The model under review builds one solid part; all positions refer to its coordinate system, in mm. Face numbers are marked on the shaded views. A direction names the side the tool comes from. Round coordinates to 2 decimals unless told otherwise and drop trailing zeros. Order: outer loops, then holes, each group sorted by start corner. A loop starts at its lowest first (then second) coordinate and runs counter-clockwise, first axis right, second up. Notation, with made-up numbers: M 79.25,37 L 124.25,37 A30 ccw 124.25,76 Z; hole C 49,68 d11. An arc over 180 degrees is marked long. Answer as a JSON object with one key per item and string values. Group by question number.
1. Mouldability with a two-part tool opening along Y and no side actions: class the marked faces 1, 2, 3 and 4 as released by +Y, released by -Y, zero draft, split by the parting line, or undercut.
2. Add section B-B on x = 32.5. State the section outline as (y, z) points (3 decimals), and give its area (3 significant figures).
3. Add section A-A on y = -14.5. State the section outline as (x, z) points, and give its area (3 significant figures).
4. Add section D-D on z = 3.25. Give the number of separate pieces and of enclosed holes in the cut face, and give its area (3 significant figures).
5. To check wall thickness, follow probe 1 along X at (y, z) = (-4, 5.25) (3 decimals); probe 2 along X at (y, z) = (8, 5.5) (3 decimals); probe 3 along Y at (x, z) = (34, 5.75) (3 decimals). State the ranges of each line that lie inside material, in increasing order. Write a range as [from, to].
6. Machinability: for the marked faces 5, 6 and 7, which of the approach directions +Z, -Z, +X, -X, +Y, -Y give a long, thin tool a straight path to every point of the face, cutting with its end or side? Answer none if there is none.
7. Add section C-C on y = -7.5. State the section outline as (x, z) points (3 decimals).
8. Clearance check with flat-ended pins moving along their axes: P1, Ø1, axis at y = -2, z = 3.5, coming from the +X side; P2, Ø1, axis at x = 27, z = 2.5, coming from the -Y side (3 decimals); P3, Ø2, axis at x = 29.5, z = 3.5, coming from the +Y side (3 decimals). State where each tip first meets the part, or that it passes through.
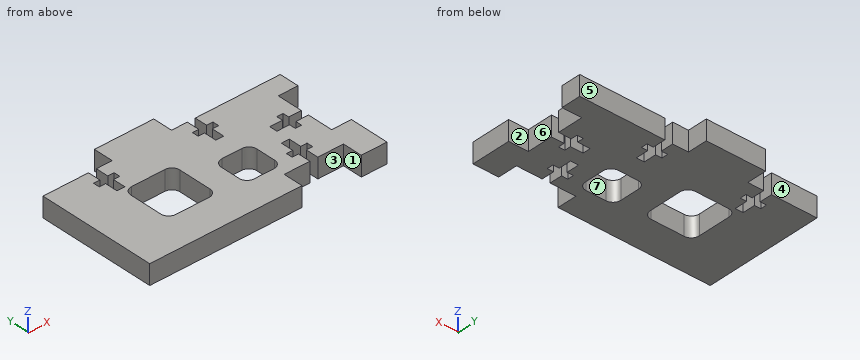
```python
from build123d import *

# Parameters (mm, degrees)
SKETCH1_W               = 76.2
SKETCH1_H               = 31.75
BOSS_EXTRUDE1_DEPTH     = 6.35
SKETCH2_W               = 19.05
SKETCH2_H               = 6.35
BOSS_EXTRUDE2_DEPTH     = 6.35
CUT_EXTRUDE1_DEPTH      = 6.35
CUT_EXTRUDE4_DEPTH      = 6.35
SKETCH5_W               = 76.2
SKETCH5_H               = 6.35
BOSS_EXTRUDE3_DEPTH     = 6.35
CUT_EXTRUDE7_DEPTH      = 1
CUT_EXTRUDE7_DEPTH_BACK = 7.35


with BuildPart() as part:
    # Sketch1 → Boss-Extrude1 (new body)
    with BuildSketch(Plane.XY):
        Rectangle(SKETCH1_W, SKETCH1_H)
    extrude(amount=BOSS_EXTRUDE1_DEPTH)

    # Sketch2 → Boss-Extrude2 (add)
    with BuildSketch(Plane.XY.offset(6.35)):
        with Locations((-6.35, 19.05)):
            Rectangle(SKETCH2_W, SKETCH2_H)
    extrude(amount=-BOSS_EXTRUDE2_DEPTH)

    # Sketch3 → Cut-Extrude1 (cut)
    with BuildSketch(Plane.XY.offset(6.35)):
        Polygon((-20.955, 11.811), (-18.923, 11.811), (-18.923, 9.779), (-20.955, 9.779), (-20.955, 5.715), (-23.495, 5.715), (-23.495, 9.779), (-25.527, 9.779), (-25.527, 11.811), (-23.495, 11.811), (-23.495, 15.875), (-20.955, 15.875), align=None)
        Polygon((8.255, 9.779), (8.255, 5.715), (10.795, 5.715), (10.795, 9.779), (12.827, 9.779), (12.827, 11.811), (10.795, 11.811), (10.795, 15.875), (8.255, 15.875), (8.255, 11.811), (6.223, 11.811), (6.223, 9.779), align=None)
    extrude(amount=-CUT_EXTRUDE1_DEPTH, mode=Mode.SUBTRACT)

    # Sketch4 → Cut-Extrude4 (cut)
    with BuildSketch(Plane.XY.offset(6.35)):
        Polygon((31.75, -9.525), (38.1, -9.525), (38.1, 9.525), (31.75, 9.525), (31.75, 1.27), (27.686, 1.27), (27.686, 3.302), (25.654, 3.302), (25.654, 1.27), (21.59, 1.27), (21.59, -1.27), (25.654, -1.27), (25.654, -3.302), (27.686, -3.302), (27.686, -1.27), (31.75, -1.27), align=None)
    extrude(amount=-CUT_EXTRUDE4_DEPTH, mode=Mode.SUBTRACT)

    # Sketch5 → Boss-Extrude3 (add)
    with BuildSketch(Plane.XY.offset(6.35)):
        with Locations((0, -19.05)):
            Rectangle(SKETCH5_W, SKETCH5_H)
    extrude(amount=-BOSS_EXTRUDE3_DEPTH)

    # Sketch8 → Cut-Extrude7 (cut, two sides)
    with BuildSketch(Plane.XY.offset(6.35)) as cut_extrude7_sk:
        with BuildLine():
            Line((-19.685, 4.699), (-9.017, 4.699))
            ThreePointArc((-9.017, 4.699), (-7.220948776, 3.955051224), (-6.477, 2.159))
            Line((-6.477, 2.159), (-6.477, -8.509))
            ThreePointArc((-6.477, -8.509), (-7.220948776, -10.305051224), (-9.017, -11.049))
            Line((-9.017, -11.049), (-19.685, -11.049))
            ThreePointArc((-19.685, -11.049), (-21.481051224, -10.305051224), (-22.225, -8.509))
            Line((-22.225, -8.509), (-22.225, 2.159))
            ThreePointArc((-22.225, 2.159), (-21.481051224, 3.955051224), (-19.685, 4.699))
        make_face()
        Polygon((10.795, -15.875), (10.795, -22.225), (29.845, -22.225), (29.845, -15.875), (21.59, -15.875), (21.59, -11.811), (23.622, -11.811), (23.622, -9.779), (21.59, -9.779), (21.59, -5.715), (19.05, -5.715), (19.05, -9.779), (17.018, -9.779), (17.018, -11.811), (19.05, -11.811), (19.05, -15.875), align=None)
        with BuildLine():
            Line((4.191, -1.0414), (10.541, -1.0414))
            ThreePointArc((10.541, -1.0414), (12.337051224, -1.785348776), (13.081, -3.5814))
            Line((13.081, -3.5814), (13.081, -9.9314))
            ThreePointArc((13.081, -9.9314), (12.337051224, -11.727451224), (10.541, -12.4714))
            Line((10.541, -12.4714), (4.191, -12.4714))
            ThreePointArc((4.191, -12.4714), (2.394948776, -11.727451224), (1.651, -9.9314))
            Line((1.651, -9.9314), (1.651, -3.5814))
            ThreePointArc((1.651, -3.5814), (2.394948776, -1.785348776), (4.191, -1.0414))
        make_face()
    extrude(amount=CUT_EXTRUDE7_DEPTH, mode=Mode.SUBTRACT)
    extrude(cut_extrude7_sk.sketch, amount=-CUT_EXTRUDE7_DEPTH_BACK, mode=Mode.SUBTRACT)


solid = part.part
```
Recorded:
{
 "1": {"face 1": "zero draft", "face 2": "undercut", "face 3": "released by -Y", "face 4": "released by +Y"},
 "2": {"outline": "M -22.225,0 L -9.525,0 L -9.525,6.35 L -22.225,6.35 Z; M 9.525,0 L 15.875,0 L 15.875,6.35 L 9.525,6.35 Z", "area": "121 mm²"},
 "3": {"outline": "M -38.1,0 L 19.05,0 L 19.05,6.35 L -38.1,6.35 Z; M 21.59,0 L 38.1,0 L 38.1,6.35 L 21.59,6.35 Z", "area": "468 mm²"},
 "4": {"separate pieces": "1", "enclosed holes": "2", "area": "2,280 mm²"},
 "5": {"probe 1": "x = [-38.1, -22.225], [-6.477, 1.651], [13.081, 31.75]", "probe 2": "x = [-38.1, -23.495], [-20.955, 8.255], [10.795, 31.75]", "probe 3": "y = [-22.225, -9.525], [9.525, 15.875]"},
 "6": {"face 5": "+Z, -Z, +X, +Y", "face 6": "+Z, -Z, +X", "face 7": "+Z, -Z"},
 "7": {"outline": "M -38.1,0 L -22.225,0 L -22.225,6.35 L -38.1,6.35 Z; M -6.477,0 L 1.651,0 L 1.651,6.35 L -6.477,6.35 Z; M 13.081,0 L 19.05,0 L 19.05,6.35 L 13.081,6.35 Z; M 21.59,0 L 31.75,0 L 31.75,6.35 L 21.59,6.35 Z"},
 "8": {"P1": "stops at x = 31.75", "P2": "stops at y = -15.875", "P3": "stops at y = 15.875"}
}
